Read the model definition and answer for the solid it produces. Units are mm, in the model's axes. Face numbers are marked on the shaded views. A direction names the side the tool comes from. Round coordinates to 2 decimals unless told otherwise and drop trailing zeros. Order: outer loops, then holes, each group sorted by start corner. A loop starts at its lowest first (then second) coordinate and runs counter-clockwise, first axis right, second up. Notation, with made-up numbers: (71.25, -36) - (106.25, -36) arc R28 cw to (106.25, -17) - close; hole circle Ø11 at (21.5, 66). An arc over 180 degrees is marked (long way). One line per question, with ' | ' between items. Start each with the question number.
1) The mould has two halves that part along Y. Classify the marked faces 1, 2, 3 and 4: pulls with the +Y half, pulls with the -Y half, needs draft (parallel to the pull), parting line crosses it, or undercut.
2) The part is cut by section C-C, the plane z = 32.5. Give the vertices of the cut face in (x, y) (3 decimals), plus the area to 3 significant figures.
3) Flat-ended cylindrical pins translate along their axes: pin 1 (8 mm diameter, centred on x = -19.05, y = 19.05, fed in from +Z); pin 2 (4 mm diameter, centred on x = 19.05, y = -19.05, fed in from -Z). Find the tip coordinate at first contact, or state that the pin passes through.
4) Straight lines are drawn through the part: line 1 (Y direction, x = -19, z = 23); line 2 (X direction, y = -16, z = 20); line 3 (Y direction, x = -21, z = 7.5). For each, find the intervals that lie inside material, in ascending order. Write a range as from..to.
5) The part is cut by section D-D, the plane z = 23. Give the vertices of the cut face in (x, y) (3 decimals).
6) The part is cut by section A-A, the plane x = 19.05. Give the vertices of the cut face in (y, z).
7) For the marked faces 5 and 6, determine the directions among +Z, -Z, +X, -X, +Y, -Y from which every point of the face is accessible in a straight line to the end or side of a thin tool.
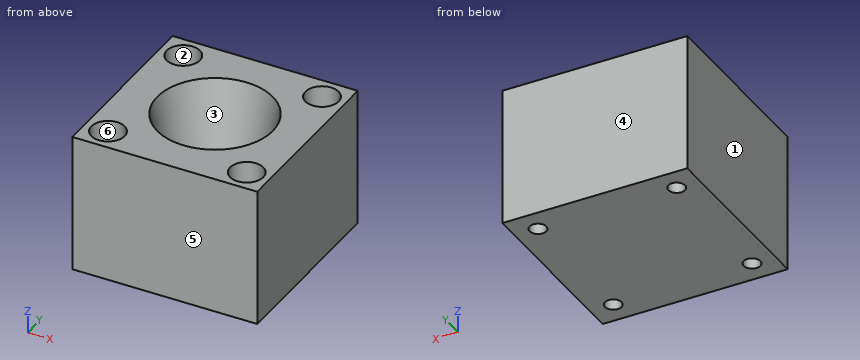
from build123d import *

# Parameters (mm, degrees)
F0_W             = 50.8
F0_H             = 50.8
F1_DEPTH         = 38.1
F2_R             = 15.875
F4_R             = 9.525
F6_R             = 4.572
F7_DEPTH         = 25.4
F9_R             = 2.286
F10_DEPTH        = 12.701
F10_COPIES_COUNT = 4


# Not quite as in the source:
# - a pattern or mirror of a feature is missing from the dataset's text; its kind, count and spacing are read off the source's solid


with BuildPart() as f1:
    # F0 (on Top) → F1 (new body)
    with BuildSketch(Plane.XY):
        Rectangle(F0_W, F0_H)
    extrude(amount=F1_DEPTH)

    # F2 (on face) → F5 section 0
    with BuildSketch(Plane.XY.offset(38.1)):
        Circle(F2_R)
    # F4 (on offset) → F5 section 1
    with BuildSketch(Plane(origin=(0, 0, 6.35), x_dir=(1, 0, 0), z_dir=(0, 0, -1))):
        Circle(F4_R)
    loft(mode=Mode.SUBTRACT)

    # F6 (on face) → F7 (cut)
    with BuildSketch(Plane.XY.offset(38.1)):
        with Locations((19.05, -19.05)):
            Circle(F6_R)
        with Locations((19.05, 19.05)):
            Circle(F6_R)
        with Locations((-19.05, 19.05)):
            Circle(F6_R)
        with Locations((-19.05, -19.05)):
            Circle(F6_R)
    extrude(amount=-F7_DEPTH, mode=Mode.SUBTRACT)

    # F9 (on offset) → F10 (cut, through all)
    with BuildSketch(Plane.XY.offset(12.7)):
        with Locations((-19.05, 19.05)):
            Circle(F9_R)
    f10 = extrude(amount=-F10_DEPTH, mode=Mode.SUBTRACT)

    # F10_copies: F10 ×4 about axis
    f10_copies_axis = Axis((0, 0, 0), (0, 0, 1))
    for i in range(1, F10_COPIES_COUNT):
        add(f10.rotate(f10_copies_axis, i * 360 / F10_COPIES_COUNT), mode=Mode.SUBTRACT)


solid = f1.part
Values:
1) face 1: needs draft | face 2: undercut | face 3: undercut | face 4: pulls with the +Y half
2) outline: (-25.4, -25.4) - (25.4, -25.4) - (25.4, 25.4) - (-25.4, 25.4) - close; hole circle Ø9.144 at (-19.05, -19.05); hole circle Ø9.144 at (-19.05, 19.05); hole circle Ø29.51 at (0, 0); hole circle Ø9.144 at (19.05, -19.05); hole circle Ø9.144 at (19.05, 19.05) | area: 1,630 mm^2
3) pin 1: stops at z = 12.7 | pin 2: passes through
4) line 1: y = -25.4..-23.62, -14.48..14.48, 23.62..25.4 | line 2: x = -25.4..-22.46, -15.64..15.64, 22.46..25.4 | line 3: y = -25.4..-20.24, -17.86..17.86, 20.24..25.4
5) outline: (-25.4, -25.4) - (25.4, -25.4) - (25.4, 25.4) - (-25.4, 25.4) - close; hole circle Ø9.144 at (-19.05, -19.05); hole circle Ø9.144 at (-19.05, 19.05); hole circle Ø25.71 at (0, 0); hole circle Ø9.144 at (19.05, -19.05); hole circle Ø9.144 at (19.05, 19.05)
6) outline: (-25.4, 0) - (-21.34, 0) - (-21.34, 12.7) - (-23.62, 12.7) - (-23.62, 38.1) - (-25.4, 38.1) - close; (-16.76, 0) - (16.76, 0) - (16.76, 12.7) - (14.48, 12.7) - (14.48, 38.1) - (-14.48, 38.1) - (-14.48, 12.7) - (-16.76, 12.7) - close; (21.34, 0) - (25.4, 0) - (25.4, 38.1) - (23.62, 38.1) - (23.62, 12.7) - (21.34, 12.7) - close
7) face 5: +Z, -Z, +X, -X, -Y | face 6: +Z
